The listing builds one solid part. Answer for the finished solid, in the listing's coordinates (mm). Face numbers are marked on the shaded views. A direction names the side the tool comes from. Coordinates: 2 decimals unless noted, no trailing zeros. Loops run counter-clockwise (first coordinate to the right, second up) from the corner with the lowest first, then second, coordinate; pieces in that order, holes last. Notation, with made-up numbers: M 31.25,30.25 L 83.25,30.25 A10 cw 83.25,40.25 Z; hole C 58.5,-38 d7. An arc over 180 degrees is marked long. Return JSON: item names as keys, results as strings. Group by question number.
1. The mould has two halves that part along Y. Classify the marked faces 1, 2 and 3: pulls with the +Y half, pulls with the -Y half, needs draft (parallel to the pull), parting line crosses it, or undercut.
2. Given P1, Ø8, axis at x = 4.5, y = -11.5, coming from the +Z side; P2, Ø4.5, axis at x = -15.5, y = -42.5, coming from the +Z side; P3, Ø4, axis at x = -6, z = 3.5, coming from the -Y side, each flat-ended and moving along its own axis, determine where each tip first touches the part or whether it passes through.
3. Which of the six approach directions +Z, -Z, +X, -X, +Y, -Y give full straight-line access (tool end or side, diameter ignored) to the marked faces 4, 5 and 6?
4. Section A-A (y = 0) is taken. Write down the section's boundary in (x, z), then the cut area to 3 significant figures.
5. Section B-B (x = 35) is taken. Write down the section's boundary in (y, z), then the cut area to 3 significant figures.
6. Section C-C (y = 42.5) is taken. Write down the section's boundary in (x, z).
7. Straight lines are drawn through the part: L1, parallel to Y at x = 17, z = 2.5; L2, parallel to Y at x = -15.5, z = 2.9; L3, parallel to Z at x = -18, y = 3.5. For each, find the intervals that lie inside material, in ascending order. Write a range as from..to.
8. Section D-D (y = -22) is taken. Write down the section's boundary in (x, z).
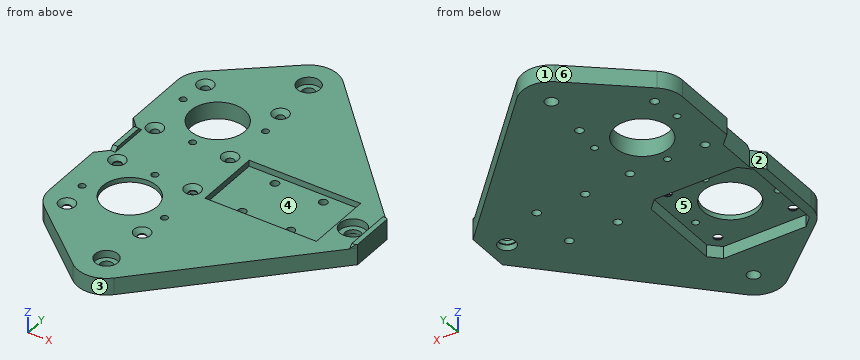
```python
from build123d import *

# Parameters (mm, degrees)
BOSS_EXTRUDE1_DEPTH                = 7
BOSS_EXTRUDE2_DEPTH                = 1.5
SKETCH29_W                         = 6.05
SKETCH29_H                         = 18.000820755
CUT_EXTRUDE6_DEPTH                 = 114.767548097
CUT_EXTRUDE1_DEPTH                 = 111.671608825
CUT_EXTRUDE1_DEPTH_BACK            = 111.671608825
SKETCH3_R                          = 11.2
CUT_EXTRUDE3_START                 = -5
CUT_EXTRUDE3_DEPTH                 = 5
SKETCH8_W                          = 46
SKETCH8_H                          = 27.2
CUT_EXTRUDE4_DEPTH                 = 2.5
CUT_EXTRUDE5_START                 = -2.4
SKETCH16_R                         = 3.6
CUT_EXTRUDE5_DEPTH                 = 2.4
CUT_EXTRUDE7_DEPTH                 = 111.776599515
SKETCH32_W                         = 1.5
SKETCH32_H                         = 16
BOSS_EXTRUDE3_DEPTH                = 2
CUT_EXTRUDE8_DEPTH                 = 129.7251141
CUT_EXTRUDE9_REACH                 = 128.86
CSK_FOR_M3_SFHCS1_D                = 3.4
CSK_FOR_M3_SFHCS1_CSINK_D          = 6.72
CSK_FOR_M3_SFHCS1_CSINK_ANGLE      = 90
M3_CLEARANCE_HOLE1_D               = 3.4
CBORE_START                        = 4
CBORE_FOR_M5_SHCS1_OUTLINE_R       = 5.4
CBORE_FOR_M5_SHCS1_DEPTH           = 3
CBORE_START_2                      = 2.4
CBORE_FOR_M5_SHCS1_2_OUTLINE_R     = 3.2
CBORE_FOR_M5_SHCS1_2_DEPTH         = 1.6
CBORE_FOR_M5_SBHCS1_OUTLINE_R      = 4.7
CBORE_FOR_M5_SBHCS1_DEPTH          = 3
CBORE_FOR_M5_SBHCS1_2_OUTLINE_R    = 2.55
CBORE_FOR_M5_SBHCS1_2_DEPTH        = 4
F_2_8_2_8_DIAMETER_HOLE1_OUTLINE_R = 1.4
F_2_8_2_8_DIAMETER_HOLE1_DEPTH     = 7


# Read off the part's stored shape, not the designer's step: CBORE for M5 SHCS1, CBORE for M5 SBHCS1, Ø2.8 (2.8) Diameter Hole1
with BuildPart() as part:
    # Sketch1 → Boss-Extrude1 (new body)
    with BuildSketch(Plane.XY):
        with BuildLine():
            Line((-25, -39.43626494), (-25, 39.43626494))
            ThreePointArc((-25, 39.43626494), (-23.875693444, 44.507684081), (-20.713451316, 48.628798257))
            Line((-20.713451316, 48.628798257), (6.236548684, 71.242533317))
            ThreePointArc((6.236548684, 71.242533317), (14.574085994, 74.03376054), (22.576586736, 70.391582661))
            Line((22.576586736, 70.391582661), (82.576586736, 8.341582661))
            ThreePointArc((82.576586736, 8.341582661), (85.95, 0), (82.576586736, -8.341582661))
            Line((82.576586736, -8.341582661), (22.576586736, -70.391582661))
            ThreePointArc((22.576586736, -70.391582661), (14.574085994, -74.03376054), (6.236548684, -71.242533317))
            Line((6.236548684, -71.242533317), (-20.713451316, -48.628798257))
            ThreePointArc((-20.713451316, -48.628798257), (-23.875693444, -44.507684081), (-25, -39.43626494))
        make_face()
    extrude(amount=BOSS_EXTRUDE1_DEPTH)

    # Sketch30 → Boss-Extrude2 (add)
    with BuildSketch(Plane.XY.offset(7)):
        with BuildLine():
            Line((79.95, 11.05791111), (79.95, -11.05791111))
            Line((79.95, -11.05791111), (82.576586736, -8.341582661))
            ThreePointArc((82.576586736, -8.341582661), (85.95, 0), (82.576586736, 8.341582661))
            Line((82.576586736, 8.341582661), (79.95, 11.05791111))
        make_face()
    extrude(amount=BOSS_EXTRUDE2_DEPTH)

    # Sketch29 → Cut-Extrude6 (cut, through all)
    with BuildSketch(Plane.XY.offset(8.5)):
        with Locations((84.975, 0.0108326)):
            Rectangle(SKETCH29_W, SKETCH29_H)
    extrude(amount=-CUT_EXTRUDE6_DEPTH, mode=Mode.SUBTRACT)

    # Sketch3 → Cut-Extrude1 (cut, two sides: drawn at the far end of the back side and taken through both)
    with BuildSketch(Plane.XY.offset(7).offset(-CUT_EXTRUDE1_DEPTH_BACK)):
        with Locations((0, 27)):
            Circle(SKETCH3_R)
        with Locations((0, -27)):
            Circle(SKETCH3_R)
    extrude(amount=CUT_EXTRUDE1_DEPTH + CUT_EXTRUDE1_DEPTH_BACK, mode=Mode.SUBTRACT)

    # Sketch6 → Cut-Extrude3 (cut)
    with BuildSketch(Plane(origin=(0, 0, 0), x_dir=(-1, 0, 0), z_dir=(0, 0, -1)).offset(CUT_EXTRUDE3_START)):
        Polygon((21.2, -9.910167799), (17.089832201, -5.8), (-17.089832201, -5.8), (-21.2, -9.910167799), (-21.2, -44.089832201), (-17.089832201, -48.2), (17.089832201, -48.2), (21.2, -44.089832201), align=None)
    extrude(amount=CUT_EXTRUDE3_DEPTH, mode=Mode.SUBTRACT)

    # Sketch8 → Cut-Extrude4 (cut)
    with BuildSketch(Plane.XY.offset(7)):
        with Locations((45, 0)):
            Rectangle(SKETCH8_W, SKETCH8_H)
    extrude(amount=-CUT_EXTRUDE4_DEPTH, mode=Mode.SUBTRACT)

    # Sketch16 → Cut-Extrude5 (cut)
    with BuildSketch(Plane(origin=(0, 0, 0), x_dir=(-1, 0, 0), z_dir=(0, 0, -1)).offset(CUT_EXTRUDE5_START)):
        with Locations((-73.95, 0)):
            Circle(SKETCH16_R)
    extrude(amount=CUT_EXTRUDE5_DEPTH, mode=Mode.SUBTRACT)

    # Sketch31 → Cut-Extrude7 (cut, through all)
    with BuildSketch(Plane(origin=(0, 0, 0), x_dir=(-1, 0, 0), z_dir=(0, 0, -1))):
        Polygon((25, -12.295954236), (20.704045764, -8), (20.704045764, 8), (25, 12.295954236), align=None)
    extrude(amount=-CUT_EXTRUDE7_DEPTH, mode=Mode.SUBTRACT)

    # Sketch32 → Boss-Extrude3 (add)
    with BuildSketch(Plane.ZY.offset(20.704045764)):
        with Locations((7.75, 0)):
            Rectangle(SKETCH32_W, SKETCH32_H)
    extrude(amount=-BOSS_EXTRUDE3_DEPTH)

    # Sketch34 → Cut-Extrude8 (cut, through all)
    with BuildSketch(Plane.ZY.offset(-79.95)):
        Polygon((7, 11.05791111), (8.5, 9.55791111), (8.5, 11.05791111), align=None)
    cut_extrude8 = extrude(amount=-CUT_EXTRUDE8_DEPTH, mode=Mode.SUBTRACT)

    # Sketch35 → Cut-Extrude9 (cut, up to next)
    with BuildSketch(Plane.ZY.offset(20.704045764), mode=Mode.PRIVATE) as cut_extrude9_sk1:
        Polygon((7, 8), (8.5, 8), (8.5, 6.5), align=None)
    cut_extrude9_tool1 = extrude(cut_extrude9_sk1.sketch, amount=-CUT_EXTRUDE9_REACH, mode=Mode.PRIVATE) & part.part
    cut_extrude9 = cut_extrude9_tool1.solids().sort_by_distance((-20.704046, 7.5, 8))[0]
    add(cut_extrude9, mode=Mode.SUBTRACT)

    # Mirror2: Cut-Extrude8, Cut-Extrude9 across plane
    add(cut_extrude8.mirror(Plane.ZX), mode=Mode.SUBTRACT)
    add(cut_extrude9.mirror(Plane.ZX), mode=Mode.SUBTRACT)

    # CSK for M3 SFHCS1 (through all)
    with Locations(Plane.XY.offset(7)):
        with Locations((-15.5, 42.5), (15.5, 42.5), (-15.5, 11.5), (15.5, -42.5), (-15.5, -42.5), (-15.5, -11.5), (15.5, 11.5), (15.5, -11.5)):
            CounterSinkHole(CSK_FOR_M3_SFHCS1_D / 2, CSK_FOR_M3_SFHCS1_CSINK_D / 2, counter_sink_angle=CSK_FOR_M3_SFHCS1_CSINK_ANGLE)

    # M3 Clearance Hole1 (through all)
    with Locations(Plane.XY.offset(4.5)):
        with Locations((35, 10), (35, -10), (55, 10), (55, -10)):
            Hole(M3_CLEARANCE_HOLE1_D / 2)

    # CBORE for M5 SHCS1 outline → CBORE for M5 SHCS1 (cut)
    with BuildSketch(Plane.XY.offset(CBORE_START)):
        with Locations((73.95, 0)):
            Circle(CBORE_FOR_M5_SHCS1_OUTLINE_R)
    extrude(amount=CBORE_FOR_M5_SHCS1_DEPTH, mode=Mode.SUBTRACT)

    # CBORE for M5 SHCS1 2 outline → CBORE for M5 SHCS1 2 (cut)
    with BuildSketch(Plane.XY.offset(CBORE_START_2)):
        with Locations((73.95, 0)):
            Circle(CBORE_FOR_M5_SHCS1_2_OUTLINE_R)
    extrude(amount=CBORE_FOR_M5_SHCS1_2_DEPTH, mode=Mode.SUBTRACT)

    # CBORE for M5 SBHCS1 outline → CBORE for M5 SBHCS1 (cut)
    with BuildSketch(Plane.XY.offset(CBORE_START)):
        with Locations((13.95, -62.05)):
            Circle(CBORE_FOR_M5_SBHCS1_OUTLINE_R)
        with Locations((13.95, 62.05)):
            Circle(CBORE_FOR_M5_SBHCS1_OUTLINE_R)
    extrude(amount=CBORE_FOR_M5_SBHCS1_DEPTH, mode=Mode.SUBTRACT)

    # CBORE for M5 SBHCS1 2 outline → CBORE for M5 SBHCS1 2 (cut)
    with BuildSketch(Plane.XY):
        with Locations((13.95, -62.05)):
            Circle(CBORE_FOR_M5_SBHCS1_2_OUTLINE_R)
        with Locations((13.95, 62.05)):
            Circle(CBORE_FOR_M5_SBHCS1_2_OUTLINE_R)
    extrude(amount=CBORE_FOR_M5_SBHCS1_2_DEPTH, mode=Mode.SUBTRACT)

    # Ø2.8 (2.8) Diameter Hole1 outline → Ø2.8 (2.8) Diameter Hole1 (cut)
    with BuildSketch(Plane.XY):
        with Locations((17, 31)):
            Circle(F_2_8_2_8_DIAMETER_HOLE1_OUTLINE_R)
        with Locations((-17, 31)):
            Circle(F_2_8_2_8_DIAMETER_HOLE1_OUTLINE_R)
        with Locations((0, 11.604631616)):
            Circle(F_2_8_2_8_DIAMETER_HOLE1_OUTLINE_R)
    f_2_8_2_8_diameter_hole1 = extrude(amount=F_2_8_2_8_DIAMETER_HOLE1_DEPTH, mode=Mode.SUBTRACT)

    # Mirror1: Ø2.8 (2.8) Diameter Hole1 across plane
    add(f_2_8_2_8_diameter_hole1.mirror(Plane.ZX), mode=Mode.SUBTRACT)


solid = part.part
```
Worked out:
{
 "1": {"face 1": "pulls with the +Y half", "face 2": "undercut", "face 3": "pulls with the -Y half"},
 "2": {"P1": "z = 7", "P2": "z = 5.89", "P3": "y = -62.65"},
 "3": {"face 4": "+Z", "face 5": "-Z", "face 6": "+Z, -Z, -X, +Y"},
 "4": {"outline": "M -20.7,0 L 70.35,0 L 70.35,2.4 L 70.75,2.4 L 70.75,4 L 68.55,4 L 68.55,7 L 68,7 L 68,4.5 L 22,4.5 L 22,7 L -18.7,7 L -18.7,8.5 L -20.7,8.5 Z; M 77.15,2.4 L 77.55,2.4 L 77.55,0 L 81.95,0 L 81.95,8.5 L 79.95,8.5 L 79.95,7 L 79.35,7 L 79.35,4 L 77.15,4 Z", "area": "550 mm^2"},
 "5": {"outline": "M -57.54,0 L -11.7,0 L -11.7,4.5 L -13.6,4.5 L -13.6,7 L -57.54,7 Z; M -8.3,0 L 8.3,0 L 8.3,4.5 L -8.3,4.5 Z; M 11.7,0 L 57.54,0 L 57.54,7 L 13.6,7 L 13.6,4.5 L 11.7,4.5 Z", "area": "707 mm^2"},
 "6": {"outline": "M -24.6,0 L -17.2,0 L -17.2,5.34 L -18.86,7 L -24.6,7 Z; M -13.8,0 L 13.8,0 L 13.8,5.34 L 12.14,7 L -12.14,7 L -13.8,5.34 Z; M 17.2,0 L 49.55,0 L 49.55,7 L 18.86,7 L 17.2,5.34 Z"},
 "7": {"L1": "-73.66..-48.2, -5.8..10.7, 12.3..29.6, 32.4..41.7, 43.3..73.66", "L2": "-53..-48.2, -5.8..9.8, 13.2..40.8, 44.2..53", "L3": "0..7"},
 "8": {"outline": "M -25,0 L -21.2,0 L -21.2,5 L -10.02,5 L -10.02,7 L -25,7 Z; M 10.02,5 L 21.2,5 L 21.2,0 L 69.37,0 L 69.37,7 L 10.02,7 Z"}
}
